```python
from build123d import *

# Parameters (mm, degrees)
F0_W     = 124.75
F0_H     = 124.75
F0_R     = 2.25
F1_DEPTH = 1
F0_W_2   = 132
F0_H_2   = 132
F2_DEPTH = 26
F4_DEPTH = 0.5
F6_DEPTH = 0.5
F7_R     = 2
F8_R     = 5


with BuildPart() as f1:
    # F0 (on Top) → F1 (new body)
    with BuildSketch(Plane.XY):
        with Locations((-0.375, 0.375)):
            Rectangle(F0_W, F0_H)
        with Locations((-33, -33)):
            Circle(F0_R, mode=Mode.SUBTRACT)
        with Locations((33, -33)):
            Circle(F0_R, mode=Mode.SUBTRACT)
        with Locations((-33, 33)):
            Circle(F0_R, mode=Mode.SUBTRACT)
        with Locations((33, 33)):
            Circle(F0_R, mode=Mode.SUBTRACT)
    extrude(amount=F1_DEPTH)

    # F0 (on Top) → F2 (join)
    with BuildSketch(Plane.XY):
        Rectangle(F0_W_2, F0_H_2)
        with Locations((-0.375, 0.375)):
            Rectangle(F0_W, F0_H, mode=Mode.SUBTRACT)
    extrude(amount=F2_DEPTH)

    # F3 (on Right) → F4 (join, symmetric)
    with BuildSketch(Plane.YZ):
        Polygon((-66, 0), (-34, 0), (-66, 8), align=None)
        Polygon((34, 0), (66, 0), (66, 8), align=None)
    extrude(amount=F4_DEPTH, both=True)

    # F5 (on Front) → F6 (join, symmetric)
    with BuildSketch(Plane.XZ):
        Polygon((-34, 0), (-66, 8), (-66, 0), align=None)
        Polygon((66, 8), (34, 0), (66, 0), align=None)
    extrude(amount=F6_DEPTH, both=True)

    # F7
    f7_edges = [f1.edges().sort_by_distance(p)[0] for p in [
        (-62.75, 62.75, 13.5),
        (62, 62.75, 13.5),
        (62, -62, 13.5),
        (-62.75, -62, 13.5),
    ]]
    fillet(f7_edges, radius=F7_R)

    # F8
    f8_edges = [f1.edges().sort_by_distance(p)[0] for p in [
        (-66, -66, 13),
        (66, -66, 13),
        (66, 66, 13),
        (-66, 66, 13),
    ]]
    fillet(f8_edges, radius=F8_R)


solid = f1.part
```
Geometry: final body of the model. Coordinates: model frame, mm. A direction names the side the tool comes from. Round coordinates to 2 decimals unless told otherwise and drop trailing zeros. Loops run counter-clockwise (first coordinate to the right, second up) from the corner with the lowest first, then second, coordinate; pieces in that order, holes last. Notation, with made-up numbers: (16, 44) -> (36, 44) arc R25 cw to (36, 57) -> close; hole circle Ø5 at (33.25, -21.5). An arc over 180 degrees is marked (long way). Use one line per item in the form item = value.
Item 1: Cut plane C-C on y = 33. Output: boundary loops of the cut face in (x, z).
Evaluation:
outline = (-66, 0) -> (-35.25, 0) -> (-35.25, 1) -> (-62.75, 1) -> (-62.75, 26) -> (-66, 26) -> close; (-30.75, 0) -> (30.75, 0) -> (30.75, 1) -> (-30.75, 1) -> close; (35.25, 0) -> (66, 0) -> (66, 26) -> (62, 26) -> (62, 1) -> (35.25, 1) -> close
Item 2: Cut plane D-D on y = 48. Output: boundary loops of the cut face in (x, z).
Evaluation:
outline = (-66, 0) -> (66, 0) -> (66, 26) -> (62, 26) -> (62, 1) -> (0.5, 1) -> (0.5, 3.5) -> (-0.5, 3.5) -> (-0.5, 1) -> (-62.75, 1) -> (-62.75, 26) -> (-66, 26) -> close
Item 3: Contact query for a flat-ended pin moving along its axis: pin 1 Ø6 at (x, y) = (-17, 6.5) entering from +Z. Output: stop coordinate, or through.
Evaluation:
pin_1 = 1
Item 4: Cut plane A-A on z = 20.75. Output: boundary loops of the cut face in (x, y).
Evaluation:
outline = (-66, -61) arc R5 ccw to (-61, -66) -> (61, -66) arc R5 ccw to (66, -61) -> (66, 61) arc R5 ccw to (61, 66) -> (-61, 66) arc R5 ccw to (-66, 61) -> close; hole (-62.75, -60) arc R2 ccw to (-60.75, -62) -> (60, -62) arc R2 ccw to (62, -60) -> (62, 60.75) arc R2 ccw to (60, 62.75) -> (-60.75, 62.75) arc R2 ccw to (-62.75, 60.75) -> close
Item 5: Cut plane B-B on x = 33. Output: boundary loops of the cut face in (y, z), then the cut area to 3 significant figures.
Evaluation:
outline = (-66, 0) -> (-35.25, 0) -> (-35.25, 1) -> (-62, 1) -> (-62, 26) -> (-66, 26) -> close; (-30.75, 0) -> (30.75, 0) -> (30.75, 1) -> (-30.75, 1) -> close; (35.25, 0) -> (66, 0) -> (66, 26) -> (62.75, 26) -> (62.75, 1) -> (35.25, 1) -> close
area = 304 mm2
Item 6: Access query for faces 4 (the cylindrical face through (-65, -64, 13)), 5 (the flat face through (-1, 1, 1)). Directions: +Z, -Z, +X, -X, +Y, -Y. A direction counts if a zero-diameter tool reaches every point of the face in a straight line with its end or side. Return the directions, or none.
Evaluation:
face_4 = +Z, -Z, -X, -Y
face_5 = +Z
Item 7: Material intervals for probe 1 along Y at (x, z) = (33, 0.8); probe 2 along Y at (x, z) = (58.5, 2.25); probe 3 along X at (y, z) = (-27, 7.5), sorted ascending.
Evaluation:
probe_1 = -66 to -35.25, -30.75 to 30.75, 35.25 to 66
probe_2 = -66 to -62, -0.5 to 0.5, 62.75 to 66
probe_3 = -66 to -62.75, 62 to 66
Item 8: Draft query along X for faces 1 (the flat face through (-66, -1, 13)), 2 (the flat face through (-1, -1, 0)), 3 (the flat face through (0.5, -56, 3)). Return one class per face: released by +X, released by -X, zero draft, split by the parting line, or undercut.
Evaluation:
face_1 = released by -X
face_2 = zero draft
face_3 = undercut
